Could you check a few things on this model? Use its own coordinates, in mm. Coordinates: 2 decimals unless noted, no trailing zeros. Loops run counter-clockwise (first coordinate to the right, second up) from the corner with the lowest first, then second, coordinate; pieces in that order, holes last.
1) Thinking about a two-plate mould opening in X: for faces 1 (the face through (-521.33, -180.99, 4.93)), 2 (the face through (-514, -166, 10)), 3 (the face through (-576.759, -187.285, 4.93)), 4 (the face through (-460.979, -167, 5)), which applies, released by +X, released by -X, zero draft, split by the parting line, or undercut?
2) Will these pins go through, and if not, where does the flat tip stop? P1, Ø2, axis at x = -574, z = 3.5, coming from the -Y side; P2, Ø4, axis at x = -561.5, z = 1.5, coming from the +Y side; P3, Ø2, axis at x = -574.5, z = 7, coming from the -Y side.
3) If I drill on line 1 along Y through (x, z) = (-574, 7.25); line 2 along X through (y, z) = (-165.5, 4.5); line 3 along X through (y, z) = (-160, 3.75), over which ranges is the centre line in solid material (lowest first)?
4) Imagine slicing it at B-B on x = -576. Please give me the cut outline in (y, z).
5) Imagine slicing it at A-A on z = 4.75. Please give me the cut outline in (x, y).
6) Imagine slicing it at C-C on y = -155. Please give me the cut outline in (x, z), plus the area to 3 significant figures.
```python
from build123d import *

# Parameters (mm, degrees)
BOSS_EXTRU_1_DEPTH = 10
D_GAGEMENT_M41_D   = 4.5


with BuildPart() as part:
    # ref externes (internes) → Boss.-Extru.1 (new body)
    with BuildSketch(Plane.XY):
        Polygon((-460.979412649, -138.268279633), (-556.886836405, -138.268279633), (-596.082218437, -179.852321051), (-556.886836405, -194.929034048), (-460.979412649, -194.929034048), align=None)
    extrude(amount=BOSS_EXTRU_1_DEPTH)

    # Dégagement M41 (through all)
    with Locations(Plane.XY.offset(10)):
        with Locations((-522.988022529, -182.510884742)):
            Hole(D_GAGEMENT_M41_D / 2)


solid = part.part
```
Filled in:
1. face 1: undercut
1. face 2: zero draft
1. face 3: released by -X
1. face 4: released by +X
2. P1: stops at y = -188.73
2. P2: stops at y = -141.04
2. P3: stops at y = -188.54
3. line 1: y = -188.35 to -156.42
3. line 2: x = -582.55 to -460.98
3. line 3: x = -577.37 to -460.98
4. outline: (-187.58, 0) - (-158.55, 0) - (-158.55, 10) - (-187.58, 10) - close
5. outline: (-596.08, -179.85) - (-556.89, -194.93) - (-460.98, -194.93) - (-460.98, -138.27) - (-556.89, -138.27) - close; hole circle Ø4.5 at (-522.99, -182.51)
6. outline: (-572.66, 0) - (-460.98, 0) - (-460.98, 10) - (-572.66, 10) - close
6. area: 1,120 mm2
